from build123d import *

# Parameters (mm, degrees)
SKETCH1_W              = 165.1
SKETCH1_H              = 127
BASE_EXTRUDE_DEPTH     = 9.525
SKETCH2_R              = 19.05
CENTER_HOLE_DEPTH      = 105.582398734
SKETCH3_W              = 50.8
SKETCH3_H              = 50.8
TOWER_EXTRUDE_DEPTH    = 63.5
FILLET_2_R             = 25.4
FILLET_2_OF_MIRROR_2_R = 25.4


with BuildPart() as part:
    # Sketch1 → Base Extrude (new body)
    with BuildSketch(Plane(origin=(0, 0, 0), x_dir=(1, 0, 0), z_dir=(0, 1, 0))):
        Rectangle(SKETCH1_W, SKETCH1_H)
    extrude(amount=BASE_EXTRUDE_DEPTH)

    # Sketch2 → Center Hole (cut, through all)
    with BuildSketch(Plane(origin=(0, 9.525, 0), x_dir=(1, 0, 0), z_dir=(0, 1, 0))):
        with Locations(Location((0, 0, 0), (0, 0, 270))):
            Circle(SKETCH2_R)
    extrude(amount=-CENTER_HOLE_DEPTH, mode=Mode.SUBTRACT)

    # Sketch3 → Tower Extrude (add)
    with BuildSketch(Plane(origin=(0, 9.525, 0), x_dir=(1, 0, 0), z_dir=(0, 1, 0))):
        with Locations((-57.15, 38.1)):
            Rectangle(SKETCH3_W, SKETCH3_H)
    tower_extrude = extrude(amount=TOWER_EXTRUDE_DEPTH)

    # Fillet 2
    fillet_2_edges = [part.edges().sort_by_distance(p)[0] for p in [
        (-31.75, 41.275, -12.7),
    ]]
    fillet(fillet_2_edges, radius=FILLET_2_R)

    # Sketch7 → 1/2-20 Tapped Hole (revolve, cut)
    with BuildSketch(Plane(origin=(-57.15, 73.025, -38.1), x_dir=(0, 0, 1), z_dir=(1, 0, 0))):
        Polygon((0, 0), (0, 35.20757432), (5.75437, 31.75), (5.75437, 0), align=None)
    f_1_2_20_tapped_hole = revolve(axis=Axis((-57.15, 79.375, -38.1), (0, -1, 0)), mode=Mode.SUBTRACT)

    # Mirror 2: Tower Extrude, 1/2-20 Tapped Hole across plane
    add(tower_extrude.mirror(Plane(origin=(0, 0, 0), x_dir=(0, 0, 1), z_dir=(1, 0, 0))))
    add(f_1_2_20_tapped_hole.mirror(Plane(origin=(0, 0, 0), x_dir=(0, 0, 1), z_dir=(1, 0, 0))), mode=Mode.SUBTRACT)

    # Fillet 2 of Mirror 2
    fillet_2_of_mirror_2_edges = [part.edges().sort_by_distance(p)[0] for p in [
        (31.75, 41.275, -12.7),
    ]]
    fillet(fillet_2_of_mirror_2_edges, radius=FILLET_2_OF_MIRROR_2_R)


solid = part.part
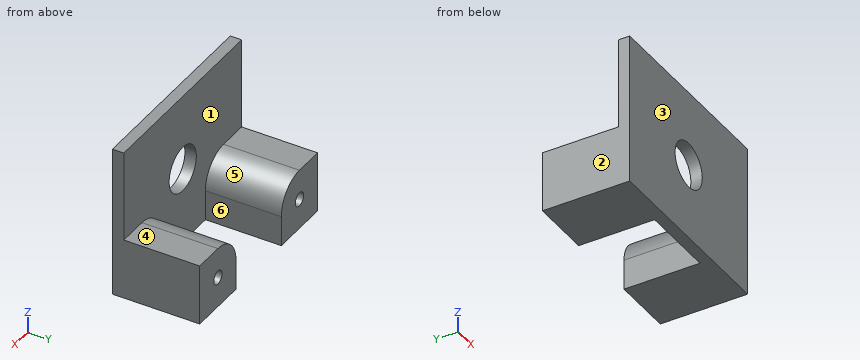
The listing builds one solid part. Answer for the finished solid, in the listing's coordinates (mm). Face numbers are marked on the shaded views. A direction names the side the tool comes from. Give positions to 0.01 mm unless a question says otherwise; leave off trailing zeros. Write each loop counter-clockwise with the first axis right and the second up, starting at its lowest first coordinate (ties: lowest second). Pieces come first, ordered by that corner, then holes.
1) Section B-B (z = 0) is taken. Write down the section's boundary in (x, y) (3 decimals), and give its area (3 significant figures).
2) Section A-A (y = 47.5) is taken. Write down the section's boundary in (x, z), and give its area (3 significant figures).
3) Find the intervals of material crossed by L1, parallel to X at y = 62, z = -38; L2, parallel to X at y = 32.5, z = -58; L3, parallel to X at y = 4, z = 0, in increasing order.
4) Section C-C (x = 0) is taken. Write down the section's boundary in (y, z) (3 decimals).
5) Given P1, Ø7.5, axis at x = 72, y = 48, coming from the +Z side; P2, Ø3, axis at x = -29.5, y = 20, coming from the +Z side, each flat-ended and moving along its own axis, determine where each tip first touches the part or whether it passes through.
6) For a pull along X with two mould halves and no side action, classify the marked faces 1, 2 and 3 as pulls with the +X half, pulls with the -X half, needs draft (parallel to the pull), parting line crosses it, or undercut.
7) Section D-D (y = 33.5) is taken. Write down the section's boundary in (x, z), and give its area (3 significant figures).
8) A tool of negligible diameter and unlimited length cuts with its end or side. For the marked faces 4, 5 and 6, from which of +Z, -Z, +X, -X, +Y, -Y can it reach the whole face along a straight path? Write none if from no direction.
Response:
1. outline: (-82.55, 0) - (-19.05, 0) - (-19.05, 9.525) - (-82.55, 9.525) - close; (19.05, 0) - (82.55, 0) - (82.55, 9.525) - (19.05, 9.525) - close
1. area: 1,210 mm2
2. outline: (-82.55, -63.5) - (-31.75, -63.5) - (-31.75, -38.1) arc R25.4 ccw to (-57.15, -12.7) - (-82.55, -12.7) - close; (31.75, -63.5) - (82.55, -63.5) - (82.55, -12.7) - (57.15, -12.7) arc R25.4 ccw to (31.75, -38.1) - close; hole circle Ø11.51 at (-57.15, -38.1); hole circle Ø11.51 at (57.15, -38.1)
2. area: 4,680 mm2
3. L1: x = -82.55 to -62.9, -51.4 to -31.75, 31.75 to 51.4, 62.9 to 82.55
3. L2: x = -82.55 to -31.75, 31.75 to 82.55
3. L3: x = -82.55 to -19.05, 19.05 to 82.55
4. outline: (0, -63.5) - (9.525, -63.5) - (9.525, -19.05) - (0, -19.05) - close; (0, 19.05) - (9.525, 19.05) - (9.525, 63.5) - (0, 63.5) - close
5. P1: stops at z = -12.7
5. P2: passes through
6. face 1: undercut
6. face 2: pulls with the -X half
6. face 3: needs draft
7. outline: (-82.55, -63.5) - (-31.75, -63.5) - (-31.75, -38.1) arc R25.4 ccw to (-57.15, -12.7) - (-82.55, -12.7) - close; (31.75, -63.5) - (82.55, -63.5) - (82.55, -12.7) - (57.15, -12.7) arc R25.4 ccw to (31.75, -38.1) - close
7. area: 4,880 mm2
8. face 4: +Z, +X, -X, +Y
8. face 5: +Z, +Y
8. face 6: +Z, -Z, +Y
